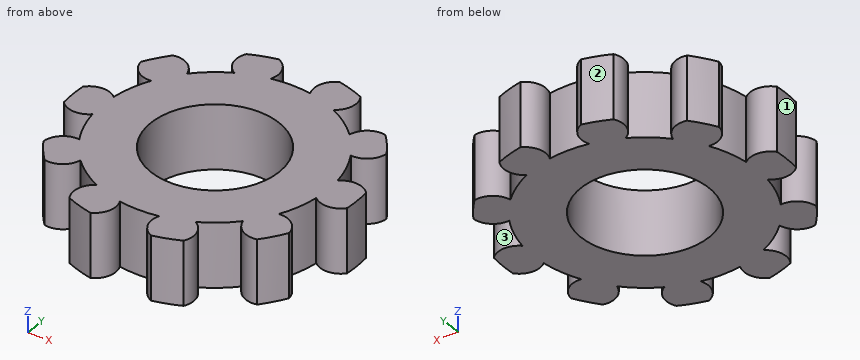
```python
from build123d import *

# Parameters (mm, degrees)
SKETCH1_R           = 13.2
SKETCH1_R_2         = 6
BOSS_EXTRUDE1_DEPTH = 6
CUT_EXTRUDE1_DEPTH  = 7
CIRPATTERN1_COUNT   = 10


with BuildPart() as part:
    # Sketch1 → Boss-Extrude1 (new body)
    with BuildSketch(Plane.XY):
        Circle(SKETCH1_R)
        Circle(SKETCH1_R_2, mode=Mode.SUBTRACT)
    extrude(amount=BOSS_EXTRUDE1_DEPTH)

    # Sketch2 → Cut-Extrude1 (cut, through all)
    with BuildSketch(Plane.XY.offset(6)):
        with BuildLine():
            ThreePointArc((-2.819851171, 12.895287487), (0, 13.2), (2.819851171, 12.895287487))
            ThreePointArc((2.819851171, 12.895287487), (1.786491669, 11.814750525), (1.819851171, 10.32))
            ThreePointArc((1.819851171, 10.32), (0, 10.479229852), (-1.819851171, 10.32))
            ThreePointArc((-1.819851171, 10.32), (-1.786491669, 11.814750525), (-2.819851171, 12.895287487))
        make_face()
    cut_extrude1 = extrude(amount=-CUT_EXTRUDE1_DEPTH, mode=Mode.SUBTRACT)

    # CirPattern1: Cut-Extrude1 ×10 about axis
    cirpattern1_axis = Axis((0, 0, 0), (0, 0, 1))
    for i in range(1, CIRPATTERN1_COUNT):
        add(cut_extrude1.rotate(cirpattern1_axis, i * 360 / CIRPATTERN1_COUNT), mode=Mode.SUBTRACT)


solid = part.part
```
For this review, take the finished solid that the model builds, in its own axes (mm). Face numbers are marked on the shaded views. Give positions to 0.01 mm unless a question says otherwise; leave off trailing zeros. Loops run counter-clockwise (first coordinate to the right, second up) from the corner with the lowest first, then second, coordinate; pieces in that order, holes last. Notation, with made-up numbers: M 30.25,27 L 86.25,27 A21 ccw 86.25,66 Z; hole C 31.5,-31.75 d2. An arc over 180 degrees is marked long. One line per item, written item: value. Start each with the question number.
Q1. Add section B-B (y = 0). Give the boundary of the cut face in (x, z), and give its area (3 significant figures).
Q2. For L1, parallel to Y at x = 0, z = 4.7; L2, parallel to X at y = -8, z = 0.95; L3, parallel to X at y = 4, z = 2.5, list the stretches that pass through material, from the lowest coordinate up.
Q3. Add section D-D (x = 7). Give the boundary of the cut face in (y, z).
Q4. Add section C-C (y = -7.75). Give the boundary of the cut face in (x, z), and give its area (3 significant figures).
Q5. Clearance check with flat-ended pins moving along their axes: pin 1 Ø2 at (x, z) = (-7.5, 2.5) entering from -Y; pin 2 Ø1.5 at (x, y) = (10.5, -5) entering from -Z; pin 3 Ø3 at (x, z) = (-0.5, 4.5) entering from +Y. State where each tip first meets the part, or that it passes through.
Q6. Add section A-A (x = 0). Give the boundary of the cut face in (y, z).
Q7. Draft analysis for pull direction Y (two halves, no side actions). For the marked faces 1, 2 and 3, state which applies: released by +Y, released by -Y, zero draft, split by the parting line, or undercut.
Reply:
1. outline: M -13.2,0 L -6,0 L -6,6 L -13.2,6 Z; M 6,0 L 13.2,0 L 13.2,6 L 6,6 Z
1. area: 86.4 mm²
2. L1: -10.48 to -6, 6 to 10.48
2. L2: -10.5 to -7.86, -6.77 to 6.77, 7.86 to 10.5
2. L3: -9.69 to -4.47, 4.47 to 9.69
3. outline: M -7.8,0 L 7.8,0 L 7.8,6 L -7.8,6 Z
4. outline: M -10.69,0 L -7.71,0 L -7.71,6 L -10.69,6 Z; M -7.05,0 L 7.05,0 L 7.05,6 L -7.05,6 Z; M 7.71,0 L 10.69,0 L 10.69,6 L 7.71,6 Z
4. area: 120 mm²
5. pin 1: y = -8.57
5. pin 2: z = 0
5. pin 3: y = 12.22
6. outline: M -10.48,0 L -6,0 L -6,6 L -10.48,6 Z; M 6,0 L 10.48,0 L 10.48,6 L 6,6 Z
7. face 1: split by the parting line
7. face 2: released by +Y
7. face 3: undercut
